```python
from build123d import *

# Parameters (mm, degrees)
SKETCH1_R           = 5.5
BOSS_EXTRUDE1_DEPTH = 20
CUT_EXTRUDE1_DEPTH  = 12
CUT_EXTRUDE2_DEPTH  = 7.8
SKETCH4_R           = 3.05
CUT_EXTRUDE3_DEPTH  = 2.3


with BuildPart() as part:
    # Sketch1 → Boss-Extrude1 (new body)
    with BuildSketch(Plane.XY):
        Circle(SKETCH1_R)
    extrude(amount=BOSS_EXTRUDE1_DEPTH)

    # Sketch2 → Cut-Extrude1 (cut)
    with BuildSketch(Plane.XY.offset(20)):
        with BuildLine():
            ThreePointArc((-1.45, -2.683281573), (3.05, 0), (-1.45, 2.683281573))
            Line((-1.45, 2.683281573), (-1.45, -2.683281573))
        make_face()
    extrude(amount=-CUT_EXTRUDE1_DEPTH, mode=Mode.SUBTRACT)

    # Sketch3 → Cut-Extrude2 (cut)
    with BuildSketch(Plane(origin=(0, 0, 0), x_dir=(-1, 0, 0), z_dir=(0, 0, -1))):
        with BuildLine():
            Line((2.3, -2.078460969), (2.3, 2.078460969))
            ThreePointArc((2.3, 2.078460969), (0, 3.1), (-2.3, 2.078460969))
            Line((-2.3, 2.078460969), (-2.3, -2.078460969))
            ThreePointArc((-2.3, -2.078460969), (0, -3.1), (2.3, -2.078460969))
        make_face()
    extrude(amount=-CUT_EXTRUDE2_DEPTH, mode=Mode.SUBTRACT)

    # Sketch4 → Cut-Extrude3 (cut)
    with BuildSketch(Plane.XY.offset(20)):
        Circle(SKETCH4_R)
    extrude(amount=-CUT_EXTRUDE3_DEPTH, mode=Mode.SUBTRACT)


solid = part.part
```
For this review, take the finished solid that the model builds, in its own axes (mm). A direction names the side the tool comes from. Round coordinates to 2 decimals unless told otherwise and drop trailing zeros. Write each loop counter-clockwise with the first axis right and the second up, starting at its lowest first coordinate (ties: lowest second). Pieces come first, ordered by that corner, then holes. Notation, with made-up numbers: M -23.75,65.5 L 34.25,65.5 A26 ccw 34.25,95.5 Z; hole C -1,-26 d3. An arc over 180 degrees is marked long. One line per item, written item: value. Start each with the question number.
(1) We need section B-B (z = 9.5). Give the boundary of the cut face in (x, y), and give its area (3 significant figures).
(2) We need section D-D (z = 18.75). Give the boundary of the cut face in (x, y), and give its area (3 significant figures).
(3) Machinability: for faces 1 (the flat face through (-3, 0, 0)), 2 (the flat face through (-2, 0, 17.7)), 3 (the flat face through (-2.3, 0, 4)), which of the approach directions +Z, -Z, +X, -X, +Y, -Y give a long, thin tool a straight path to every point of the face, cutting with its end or side? Answer none if there is none.
(4) Insertion check: pin 1 (1.3 mm diameter, centred on x = -2, y = 1, fed in from +Z); pin 2 (2.5 mm diameter, centred on x = 1, y = -1.5, fed in from -Z); pin 3 (1.5 mm diameter, centred on y = -2, z = 12.5, fed in from -X). Each pin has a flat end and moves straight along its axis. Give the tip position at first contact, or say it passes through.
(5) We need section C-C (x = 0). Give the boundary of the cut face in (y, z), and give its area (3 significant figures).
(6) We need section A-A (y = 0). Give the boundary of the cut face in (x, z).
(7) The part is to be moulded in two halves that separate along X. For faces 4 (the cylindrical face through (0, 3.1, 3.8)), 5 (the cylindrical face through (-1.19, -5.37, 9.86)), 6 (the flat face through (2.4, -2.4, 20)), say which applies: released by +X, released by -X, zero draft, split by the parting line, or undercut.
(8) Wall thickness on line 1 (Y direction, x = 0, z = 11.25); line 2 (Z direction, x = -1, y = -0.5); line 3 (X direction, y = 2.5, z = 9.5): over which ranges is each line inside the solid? List them lowest first.
Result:
1. outline: C 0,0 d11; hole M -1.45,-2.68 A3.05 ccw long -1.45,2.68 Z
1. area: 71.9 mm²
2. outline: C 0,0 d11; hole C 0,0 d6.1
2. area: 65.8 mm²
3. face 1: -Z, +X, -X, +Y, -Y
3. face 2: +Z
3. face 3: -Z
4. pin 1: z = 17.7
4. pin 2: z = 7.8
4. pin 3: x = -5.36
5. outline: M -5.5,0 L -3.1,0 L -3.1,7.8 L 3.1,7.8 L 3.1,0 L 5.5,0 L 5.5,20 L 3.05,20 L 3.05,8 L -3.05,8 L -3.05,20 L -5.5,20 Z
5. area: 98.4 mm²
6. outline: M -5.5,0 L -2.3,0 L -2.3,7.8 L 2.3,7.8 L 2.3,0 L 5.5,0 L 5.5,20 L 3.05,20 L 3.05,8 L -1.45,8 L -1.45,17.7 L -3.05,17.7 L -3.05,20 L -5.5,20 Z
7. face 4: undercut
7. face 5: split by the parting line
7. face 6: zero draft
8. line 1: -5.5 to -3.05, 3.05 to 5.5
8. line 2: 7.8 to 8
8. line 3: -4.9 to -1.45, 1.75 to 4.9
